Input: part model. Units: mm. Frame: model coordinates. Face numbers are marked on the shaded views. A direction names the side the tool comes from. Give positions to 0.01 mm unless a question says otherwise; leave off trailing zeros. Write each loop counter-clockwise with the first axis right and the second up, starting at its lowest first coordinate (ties: lowest second). Pieces come first, ordered by that corner, then holes. Notation, with made-up numbers: (31, -28.75) -> (55, -28.75) arc R27 cw to (55, -6.75) -> close; hole circle Ø1 at (45, 40). An arc over 180 degrees is marked (long way). Return JSON: item names as keys, results as strings. Group by question number.
Item 1: Section A-A, the plane x = 0. Return loops of the section in (y, z).
Item 2: Set-up query: the marked faces 4 and 5. Return all of +Z, -Z, +X, -X, +Y, -Y with unobstructed straight access to the full face (end or side cutting, diameter ignored); none if empty.
Item 3: Mould query, pull axis Y, two halves, no side actions, for the marked faces 1, 2 and 3. Classes: released by +Y, released by -Y, zero draft, split by the parting line, or undercut.
Item 4: Line query: line 1 (X direction, y = 0, z = 0.6); line 2 (Y direction, x = 0, z = 0.6); line 3 (X direction, y = 0, z = 0.3). Output: solid intervals per line, ascending. Write a range as [from, to].
Item 5: Pin query (flat end, axial travel): P1, Ø1.6, axis at y = -4.5, z = 1.5, coming from the +X side; P2, Ø10, axis at x = -2, y = 5.5, coming from the +Z side; P3, Ø0.9, axis at x = -9.5, y = 1.5, coming from the -Z side. Return the tip coordinate at first contact, or that it passes through.
from build123d import *

# Parameters (mm, degrees)
F3_DEPTH  = 0.35
F4_DEPTH  = 5
F5_W      = 3.3258799294
F5_H      = 4.7764119825
F6_DEPTH  = 6
F8_START  = 1
F7_W      = 3
F7_H      = 20.7612029826
F8_DEPTH  = 2
F12_DEPTH = 2.9


with BuildPart() as f1:
    # F0 (on Front) → F1 (revolve)
    with BuildSketch(Plane.XZ):
        Polygon((-6, 1), (-12, 3), (-16.4613984525, 3), (-17, 3), (-17, 0), (-6, 0), align=None)
        Polygon((-17, 3), (-16.4613984525, 3), (-17, 3.4264510032), align=None)
    revolve(axis=Axis((0, 0, 0.3460962325), (0, 0, -1)))

    # F2 (on Top) → F3 (cut)
    with BuildSketch(Plane.XY):
        with BuildLine():
            Line((12.9273881117, 1), (2.0039374787, 5.6685529396))
            Line((2.0039374787, 5.6685529396), (2.0039374787, -5.6685529396))
            Line((2.0039374787, -5.6685529396), (12.9273881117, -1))
            ThreePointArc((12.9273881117, -1), (13.5875019991, 0), (12.9273881117, 1))
        make_face()
    extrude(amount=F3_DEPTH, mode=Mode.SUBTRACT)

    # F2 (on Top) → F4 (cut)
    with BuildSketch(Plane.XY):
        with BuildLine():
            Line((-2.0039374787, -5.6685529396), (-2.0039374787, 5.6685529396))
            Line((-2.0039374787, 5.6685529396), (-12.9273881117, 1))
            ThreePointArc((-12.9273881117, 1), (-13.5875019991, 0), (-12.9273881117, -1))
            Line((-12.9273881117, -1), (-2.0039374787, -5.6685529396))
        make_face()
    extrude(amount=F4_DEPTH, mode=Mode.SUBTRACT)

    # F5 (on Top) → F6 (join)
    with BuildSketch(Plane.XY):
        with Locations((-15.1684732898, 0)):
            Rectangle(F5_W, F5_H)
        with Locations((15.1684732898, 0)):
            Rectangle(F5_W, F5_H)
    extrude(amount=F6_DEPTH)

    # F7 (on Top) → F8 (join)
    with BuildSketch(Plane.XY.offset(F8_START)):
        with Locations((-9, 0)):
            Rectangle(F7_W, F7_H)
    extrude(amount=F8_DEPTH)

    # F9 (on Front) → F10 (revolve, cut)
    with BuildSketch(Plane.XZ):
        Polygon((8.2996124042, 0.1023378446), (9, 0), (16.3225417007, 5.4439346324), (15.9651809612, 5.801295372), align=None)
        Polygon((15.9651809612, 5.801295372), (16.3225417007, 5.4439346324), (17.0113109052, 5.9559992515), (16.7064689267, 6.3524049994), align=None)
    revolve(axis=Axis((13.0056554526, 0, 2.9779996257), (0.802516509, 0, 0.5966299128)), mode=Mode.SUBTRACT)

    # F9 (on Front) → F11 (revolve, cut)
    with BuildSketch(Plane.XZ):
        Polygon((-16.7743696364, 6.1416257066), (-17.127923027, 5.7880723161), (-16.5531635221, 5.2133128111), (-16.1996101315, 5.5668662017), align=None)
        Polygon((-16.1996101315, 5.5668662017), (-16.5531635221, 5.2133128111), (-12.5092434766, 1.1693927656), (-12.155690086, 1.5229461562), align=None)
    revolve(axis=Axis((-14.4650298612, 0, 3.8322859314), (-0.7071067812, 0, 0.7071067812)), mode=Mode.SUBTRACT)

    # F9 (on Front) → F12 (cut, symmetric)
    with BuildSketch(Plane.XZ):
        Polygon((-16.5531635221, 5.2133128111), (-17.127923027, 5.7880723161), (-16.7743696364, 6.1416257066), (-16.1996101315, 5.5668662017), (-15.1436466258, 6.6228297073), (-17.0755104627, 8.5546935443), (-19.2268886647, 6.4033153423), (-17.2588344452, 4.507641888), align=None)
        Polygon((-16.7743696364, 6.1416257066), (-17.127923027, 5.7880723161), (-16.5531635221, 5.2133128111), (-16.1996101315, 5.5668662017), align=None)
        Polygon((15.9651809612, 5.801295372), (16.3225417007, 5.4439346324), (17.0113109052, 5.9559992515), (16.7064689267, 6.3524049994), align=None)
        Polygon((17.0113109052, 5.9559992515), (16.3225417007, 5.4439346324), (17.2588344452, 4.507641888), (19.2268886647, 6.4033153423), (17.0755104627, 8.5546935443), (15.1436466258, 6.6228297073), (15.9651809612, 5.801295372), (16.7064689267, 6.3524049994), align=None)
    extrude(amount=F12_DEPTH, both=True, mode=Mode.SUBTRACT)


solid = f1.part
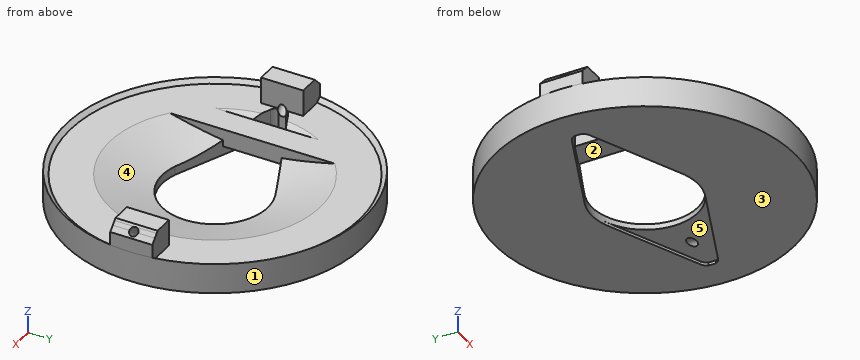
Answer below:
{
 "1": {"outline": "(-17, 0) -> (-6, 0) -> (-6, 1) -> (-12, 3) -> (-16.46, 3) -> (-17, 3.43) -> close; (6, 0) -> (17, 0) -> (17, 3.43) -> (16.46, 3) -> (12, 3) -> (6, 1) -> close"},
 "2": {"face 4": "+Z", "face 5": "-Z"},
 "3": {"face 1": "split by the parting line", "face 2": "undercut", "face 3": "zero draft"},
 "4": {"line 1": "x = [-17, -13.51], [6, 8.97], [10.65, 17]", "line 2": "y = [-17, -6], [6, 17]", "line 3": "x = [-17, -13.51], [13.51, 17]"},
 "5": {"P1": "stops at x = 16.59", "P2": "stops at z = 2.62", "P3": "stops at z = 1"}
}
